Part model, mm, in its own coordinate system. A direction names the side the tool comes from. Coordinates: 2 decimals unless noted, no trailing zeros. Loops run counter-clockwise (first coordinate to the right, second up) from the corner with the lowest first, then second, coordinate; pieces in that order, holes last. Notation, with made-up numbers: M 12,-11 L 57,-11 A29 ccw 57,10 Z; hole C 31,24.25 d3. An arc over 180 degrees is marked long. Answer as a JSON object with one key per item and string values. Group by question number.
1. Mould opens along Y. For faces 1 (the face through (15.12, -17.826, 1.479)), 2 (the face through (30.35, 0.08, 1.48)), 3 (the face through (-22.324, -14, 1)), 4 (the face through (-11.25, -17.28, 1.48)) say: released by +Y, released by -Y, zero draft, split by the parting line, or undercut.
2. Saw through at B-B on z = 0.9. Write the cut outline in (x, y), then the cut area to 3 significant figures.
3. 3-axis set-ups, long thin cutter, end or side, ignore diameter. For faces 5 (the face through (-12, -27.967, 1)), 6 (the face through (-2.324, -19, 1)), 7 (the face through (-10.417, -6.366, 1.479)): which of +Z, -Z, +X, -X, +Y, -Y reach the whole face in a straight line?
4. Saw through at A-A on x = -17. Write the cut outline in (y, z).
5. Saw through at C-C on y = 5. Write the cut outline in (x, z), then the cut area to 3 significant figures.
6. Saw through at D-D on x = -7. Write the cut outline in (y, z), then the cut area to 3 significant figures.
7. Drill centre lines: L1, parallel to Y at x = -12.5, z = 1.8; L2, parallel to X at y = -15, z = 0.6; L3, parallel to X at y = -20.5, z = 0.45. Where is each one in solid material? Low to high.
8. Drop flat-ended pins along their axis: pin 1 Ø3 at (x, y) = (-2.32, 12.03) entering from -Z; pin 2 Ø0.9 at (x, z) = (-11.5, 1.5) entering from -Y. Give the stop position or say it passes through.
from build123d import *

# Parameters (mm, degrees)
SKETCH_1_R      = 2
EXTRUDE_1_DEPTH = 3


with BuildPart() as part:
    # 草图1 → 凸台-拉伸1 (new body)
    with BuildSketch(Plane.XY):
        with BuildLine():
            Line((-22.324440756, -1.353097581), (-22.324440756, -27.966719239))
            Line((-22.324440756, -27.966719239), (-2.324440756, -27.966719239))
            Line((-2.324440756, -27.966719239), (-2.324440756, -10.197546911))
            ThreePointArc((-2.324440756, -10.197546911), (-0.7958984, -7.583199497), (2.232100844, -7.632945919))
            ThreePointArc((2.232100844, -7.632945919), (15.283597331, -17.99273018), (25.355051168, -31.267989428))
            Line((25.355051168, -31.267989428), (42.675559244, -21.267989428))
            Line((42.675559244, -21.267989428), (17.675559244, 22.033280761))
            Line((17.675559244, 22.033280761), (-32.324440756, 22.033280761))
            Line((-32.324440756, 22.033280761), (-32.324440756, 2.033280761))
            ThreePointArc((-32.324440756, 2.033280761), (-28.653774048, 1.932053083), (-24.994265265, 1.628677754))
            ThreePointArc((-24.994265265, 1.628677754), (-23.089432202, 0.64808626), (-22.324440756, -1.353097581))
        make_face()
        with Locations((-17.324440756, 12.033280761)):
            Circle(SKETCH_1_R, mode=Mode.SUBTRACT)
        with Locations((-2.324440756, 12.033280761)):
            Circle(SKETCH_1_R, mode=Mode.SUBTRACT)
        with Locations((19.015305206, -0.287227314)):
            Circle(SKETCH_1_R, mode=Mode.SUBTRACT)
        with Locations((26.515305206, -13.277608371)):
            Circle(SKETCH_1_R, mode=Mode.SUBTRACT)
        with Locations((-12.324440756, -18.966719239)):
            Circle(SKETCH_1_R, mode=Mode.SUBTRACT)
        with Locations((-12.324440756, -6.966719239)):
            Circle(SKETCH_1_R, mode=Mode.SUBTRACT)
    extrude(amount=EXTRUDE_1_DEPTH)


solid = part.part
Outcome:
{
 "1": {"face 1": "released by -Y", "face 2": "released by +Y", "face 3": "zero draft", "face 4": "undercut"},
 "2": {"outline": "M -32.32,2.03 A66.6 cw -24.99,1.63 A3 cw -22.32,-1.35 L -22.32,-27.97 L -2.32,-27.97 L -2.32,-10.2 A3 cw 2.23,-7.63 A66.6 cw 25.36,-31.27 L 42.68,-21.27 L 17.68,22.03 L -32.32,22.03 Z; hole C -17.32,12.03 d4; hole C -12.32,-18.97 d4; hole C -12.32,-6.97 d4; hole C -2.32,12.03 d4; hole C 19.02,-0.29 d4; hole C 26.52,-13.28 d4", "area": "2,470 mm²"},
 "3": {"face 5": "+Z, -Z, -X, -Y", "face 6": "+Z, -Z, -Y", "face 7": "+Z, -Z"},
 "4": {"outline": "M -27.97,0 L 10.06,0 L 10.06,3 L -27.97,3 Z; M 14.01,0 L 22.03,0 L 22.03,3 L 14.01,3 Z"},
 "5": {"outline": "M -32.32,0 L 27.51,0 L 27.51,3 L -32.32,3 Z", "area": "180 mm²"},
 "6": {"outline": "M -27.97,0 L 22.03,0 L 22.03,3 L -27.97,3 Z", "area": "150 mm²"},
 "7": {"L1": "y = -27.97 to -20.96, -16.97 to -8.96, -4.97 to 22.03", "L2": "x = -22.32 to -2.32, 12.16 to 25.5, 27.53 to 39.06", "L3": "x = -22.32 to -13.61, -11.04 to -2.32, 17.61 to 42.23"},
 "8": {"pin 1": "passes through", "pin 2": "stops at y = -27.97"}
}
